```python
from build123d import *

# Parameters (mm, degrees)
F0_W     = 12.8171369433
F0_H     = 152.6404321194
F0_R     = 1.9711085463
F1_DEPTH = 6.35
F2_W     = 12.8171369433
F2_H     = 6.35
F2_W_2   = 16.510868445
F2_W_3   = 16.5063254535
F3_DEPTH = 1.27
F4_R     = 2.9604656486
F4_R_2   = 2.9553822982
F5_DEPTH = 1.27
F5_TAPER = 35


with BuildPart() as f1:
    # F0 (on Top) → F1 (new body)
    with BuildSketch(Plane.XY):
        Rectangle(F0_W, F0_H)
        with Locations((0, -67.9932013154)):
            Circle(F0_R, mode=Mode.SUBTRACT)
    extrude(amount=F1_DEPTH)

    # F2 (on face) → F3 (join)
    with BuildSketch(Plane(origin=(0, 76.3202160597, 0), x_dir=(-1, 0, 0), z_dir=(0, 1, 0))):
        with Locations((0, 3.175)):
            Rectangle(F2_W, F2_H)
        with Locations((-14.6640026942, 3.175)):
            Rectangle(F2_W_2, F2_H)
        with Locations((14.6617311984, 3.175)):
            Rectangle(F2_W_3, F2_H)
        Polygon((6.4085684717, 0), (-6.4085684717, 0), (-22.9194369167, 0), (-22.9194369167, -12.6968417317), (22.9148939252, -12.6968417317), (22.9148939252, 0), align=None)
    extrude(amount=F3_DEPTH)

    # F4 (on face) → F5 (cut)
    with BuildSketch(Plane.XZ.offset(-76.3202160597)):
        with Locations((11.4597184584, -6.3484208658)):
            Circle(F4_R)
        with Locations((-11.4574469626, -6.3484208658)):
            Circle(F4_R_2)
    extrude(amount=-F5_DEPTH, taper=F5_TAPER, mode=Mode.SUBTRACT)


solid = f1.part
```
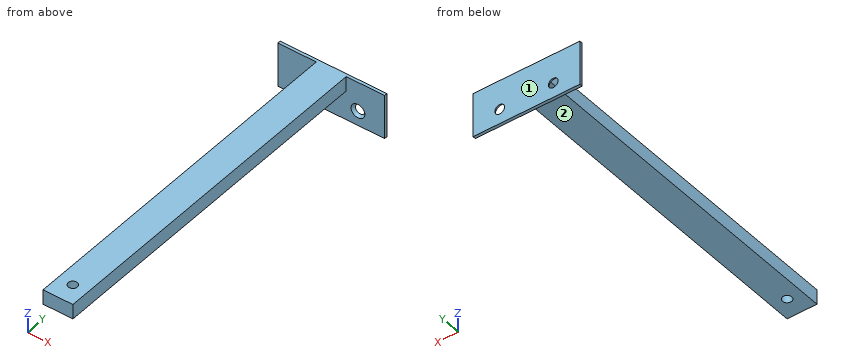
Part model, mm, in its own coordinate system. Face numbers are marked on the shaded views. A direction names the side the tool comes from. Round coordinates to 2 decimals unless told otherwise and drop trailing zeros. Loops run counter-clockwise (first coordinate to the right, second up) from the corner with the lowest first, then second, coordinate; pieces in that order, holes last.
1. Flat gauge pins, fed straight in: pin 1 (7 mm diameter, centred on y = -18, z = 4.5, fed in from +X); pin 2 (6.5 mm diameter, centred on x = 0, y = 6, fed in from -Z); pin 3 (8 mm diameter, centred on x = 1, z = -10, fed in from -Y). Where does each tip first touch, or does it go through?
Solutions:
pin 1: stops at x = 6.41
pin 2: stops at z = 0
pin 3: stops at y = 76.32
2. Drill centre lines: line 1 along Y through (x, z) = (0, 4.75); line 2 along X through (y, z) = (66, 3.75); line 3 along Y through (x, z) = (11, 3.5). Where is each one in solid material? Low to high.
Solutions:
line 1: y = -76.32 to -69.96, -66.02 to 77.59
line 2: x = -6.41 to 6.41
line 3: y = 76.32 to 77.59
3. 3-axis set-ups, long thin cutter, end or side, ignore diameter. For the marked faces 1 and 2: which of +Z, -Z, +X, -X, +Y, -Y reach the whole face in a straight line?
Solutions:
face 1: +Z, -Z, +X, -X, +Y
face 2: -Z, +X, -X, -Y
4. Slice it at A-A (x = 0). Give the cut face in (y, z).
Solutions:
outline: (-76.32, 0) - (-69.96, 0) - (-69.96, 6.35) - (-76.32, 6.35) - close; (-66.02, 0) - (76.32, 0) - (76.32, -12.7) - (77.59, -12.7) - (77.59, 6.35) - (-66.02, 6.35) - close
5. Slice it at B-B (z = 3). Give the cut face in (x, y), and give its area (3 significant figures).
Solutions:
outline: (-22.91, 76.32) - (-6.41, 76.32) - (-6.41, -76.32) - (6.41, -76.32) - (6.41, 76.32) - (22.92, 76.32) - (22.92, 77.59) - (-22.91, 77.59) - close; hole circle Ø3.94 at (0, -67.99)
area: 2,000 mm2
6. Slice it at C-C (y = -52.5). Give the cut face in (x, z).
Solutions:
outline: (-6.41, 0) - (6.41, 0) - (6.41, 6.35) - (-6.41, 6.35) - close
